Input: part model. Units: mm. Frame: model coordinates. Face numbers are marked on the shaded views. Coordinates: 2 decimals unless noted, no trailing zeros. Write each loop counter-clockwise with the first axis right and the second up, starting at its lowest first coordinate (ties: lowest second). Pieces come first, ordered by that corner, then holes. Notation, with made-up numbers: M 40,29 L 77,29 A26 ccw 77,43 Z; hole C 44,11.25 d2. An arc over 180 degrees is marked long. Write each question's results on one line, items separated by ' | '. Start each with the question number.
1. Pull-direction query (Y, two-part tool) for the marked faces 1, 2 and 3; classes: +Y half, -Y half, draft (parallel to the pull), parting line (faces both ways), or undercut.
2. First-contact query: pin 1 (8 mm diameter, centred on x = 440.5, y = 47, fed in from +Z). Flat tip, straight axial feed; report the tip coordinate or a pass-through.
3. Section query B-B, the plane x = 404.5. Output: boundary loops of the cut face in (y, z), and give its area (3 significant figures).
4. Ray query, probe 1 along Y at (x, z) = (378, 28.5); probe 2 along Z at (x, y) = (453.5, 60). Return the intervals inside material, ascending.
5. Section query A-A, the plane y = 41. Output: boundary loops of the cut face in (x, z), and give its area (3 significant figures).
```python
from build123d import *

# Parameters (mm, degrees)
CEK_DONMUS_ON_PU_37_5_1_START = 1
SKETCH1_W                     = 618
SKETCH1_H                     = 88
CEK_DONMUS_ON_PU_37_5_1_DEPTH = 37.5
CEK_DONMUS_ON_PU_37_5_2_START = 27
SKETCH2_W                     = 300
SKETCH2_H                     = 34
CEK_DONMUS_ON_PU_37_5_2_DEPTH = 14


with BuildPart() as part:
    # Sketch1 → CEK_donmus_on_pu_37.5_1 (new body)
    with BuildSketch(Plane.XY.offset(CEK_DONMUS_ON_PU_37_5_1_START)):
        with Locations((309, 44)):
            Rectangle(SKETCH1_W, SKETCH1_H)
    extrude(amount=CEK_DONMUS_ON_PU_37_5_1_DEPTH)

    # Sketch2 → CEK_donmus_on_pu_37.5_2 (cut)
    with BuildSketch(Plane.XY.offset(CEK_DONMUS_ON_PU_37_5_2_START)):
        with Locations((309, 45)):
            Rectangle(SKETCH2_W, SKETCH2_H)
    extrude(amount=CEK_DONMUS_ON_PU_37_5_2_DEPTH, mode=Mode.SUBTRACT)


solid = part.part
```
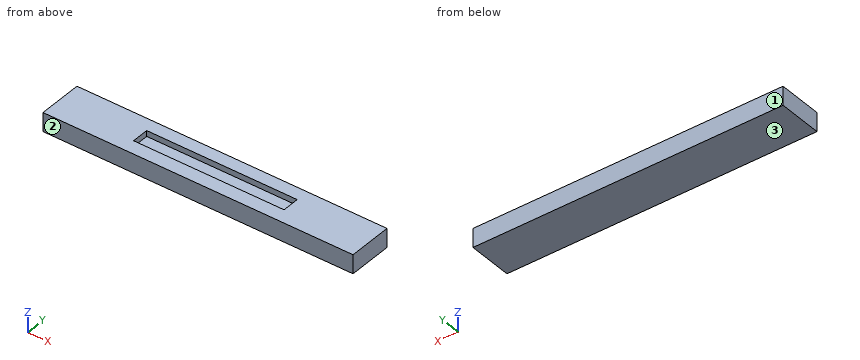
Answer:
1) face 1: +Y half | face 2: -Y half | face 3: draft
2) pin 1: z = 27
3) outline: M 0,1 L 88,1 L 88,38.5 L 62,38.5 L 62,27 L 28,27 L 28,38.5 L 0,38.5 Z | area: 2,910 mm^2
4) probe 1: 0 to 28, 62 to 88 | probe 2: 1 to 27
5) outline: M 0,1 L 618,1 L 618,38.5 L 459,38.5 L 459,27 L 159,27 L 159,38.5 L 0,38.5 Z | area: 19,700 mm^2
